Input: part model. Units: mm. Frame: model coordinates. A direction names the side the tool comes from. Give positions to 0.01 mm unless a question says otherwise; leave off trailing zeros. Loops run counter-clockwise (first coordinate to the right, second up) from the corner with the lowest first, then second, coordinate; pieces in that order, holes last. Notation, with made-up numbers: (42.5, 61.5) - (96.5, 61.5) arc R15 cw to (96.5, 69.5) - close; hole circle Ø4 at (9.25, 80.5). An arc over 180 degrees is marked (long way). Answer as a JSON object with one key per item and string values. Group by question number.
(1) Access query for faces 1 (the cylindrical face through (14.13, 1.69, 1.84)), 2 (the flat face through (4.06, -6.66, 5.94)), 3 (the flat face through (4.06, 6.66, -5.94)). Directions: +Z, -Z, +X, -X, +Y, -Y. A direction counts if a zero-diameter tool reaches every point of the face in a straight line with its end or side. Return the directions, or none.
(2) Section query B-B (x = 21). Return loops of the section in (y, z), plus the area to 3 significant figures.
(3) Pin query (flat end, axial travel): P1, Ø4, axis at x = 4, z = 1.5, coming from the -Y side; P2, Ø3.5, axis at y = -0.5, z = -0.5, coming from the +X side; P3, Ø6, axis at x = 17, z = 7.5, coming from the -Y side. Return the tip coordinate at first contact, or that it passes through.
(4) Mould query, pull axis X, two halves, no side actions, for faces 4 (the cylindrical face through (17.666, -8.428, -1.107)), 5 (the flat face through (23, -2, -2)), 6 (the flat face through (13.209, -7, 3)), 7 (the flat face through (0, 0, 0)). Classes: +X half, -X half, draft (parallel to the pull), parting line (faces both ways), or undercut.
(5) Material intervals for L1, parallel to Y at x = 17.75, z = 0; L2, parallel to Y at x = 10.5, z = 0; L3, parallel to X at y = -11, z = 6.75, sorted ascending.
(6) Section query A-A (x = 7.5). Return loops of the section in (y, z).
```python
from build123d import *

# Parameters (mm, degrees)
EXTRUDE_START            = -8
SKETCH_2_R               = 8.5
EXTRUDE_1_DEPTH          = 8
CHAMFER_1_SIZE           = 1
SKETCH_3_R               = 2.5
CUT_EXTRUDE_1_DEPTH      = 18
CUT_EXTRUDE_2_DEPTH      = 18
CUT_EXTRUDE_2_DEPTH_BACK = 8.454068
SKETCH_4_R               = 2.5


with BuildPart() as part:
    # Sketch 1 → 旋转1 (revolve)
    with BuildSketch(Plane.XY, mode=Mode.PRIVATE) as revolve_1_sk:
        Polygon((0, 0), (0, 8.5), (8, 8.5), (8, 13), (11, 13), (11.209265355, 7.3), (13.209265355, 7.3), (13.209265355, 8.5), (23, 8.5), (23, 0), align=None)
    revolve(revolve_1_sk.sketch.rotate(Axis((0, 0, 0), (1, 0, 0)), 90), axis=Axis((0, 0, 0), (1, 0, 0)))

    # 草图2 → 凸台-拉伸1 (add)
    # profile 1 of 7: a face of its own
    with BuildSketch(Plane.ZY.offset(EXTRUDE_START)):
        Polygon((-1.174764966, -9.690972033), (7.805245485, -5.86286232), (8.980010451, 3.828109713), (1.174764966, 9.690972033), (-7.805245485, 5.86286232), (-8.980010451, -3.828109713), align=None)
        Circle(SKETCH_2_R, mode=Mode.SUBTRACT)
    # profile 2 of 7: a face of its own
    with BuildSketch(Plane.ZY.offset(EXTRUDE_START)):
        with BuildLine():
            Line((-7.805245485, 5.86286232), (-8.286430908, 1.893426207))
            ThreePointArc((-8.286430908, 1.893426207), (-6.796266629, 5.104974035), (-4.12702026, 7.430861577))
            Line((-4.12702026, 7.430861577), (-7.805245485, 5.86286232))
        make_face()
    # profile 3 of 7: a face of its own
    with BuildSketch(Plane.ZY.offset(EXTRUDE_START)):
        with BuildLine():
            ThreePointArc((-2.503460259, 8.122972777), (1.022903886, 8.43822657), (4.371804767, 7.289535176))
            Line((4.371804767, 7.289535176), (1.174764966, 9.690972033))
            Line((1.174764966, 9.690972033), (-2.503460259, 8.122972777))
        make_face()
    # profile 4 of 7: a face of its own
    with BuildSketch(Plane.ZY.offset(EXTRUDE_START)):
        with BuildLine():
            ThreePointArc((8.5, 0), (8.499706252, -0.070665642), (8.498825028, -0.141326401))
            Line((8.498825028, -0.141326401), (8.980010451, 3.828109713))
            Line((8.980010451, 3.828109713), (5.78297065, 6.22954657))
            ThreePointArc((5.78297065, 6.22954657), (7.79118895, 3.398142837), (8.5, 0))
        make_face()
    # profile 5 of 7: a face of its own
    with BuildSketch(Plane.ZY.offset(EXTRUDE_START)):
        with BuildLine():
            Line((4.12702026, -7.430861577), (7.805245485, -5.86286232))
            Line((7.805245485, -5.86286232), (8.286430908, -1.893426207))
            ThreePointArc((8.286430908, -1.893426207), (6.796266629, -5.104974035), (4.12702026, -7.430861577))
        make_face()
    # profile 6 of 7: a face of its own
    with BuildSketch(Plane.ZY.offset(EXTRUDE_START)):
        with BuildLine():
            Line((-1.174764966, -9.690972033), (2.503460259, -8.122972777))
            ThreePointArc((2.503460259, -8.122972777), (-1.022903886, -8.43822657), (-4.371804767, -7.289535176))
            Line((-4.371804767, -7.289535176), (-1.174764966, -9.690972033))
        make_face()
    # profile 7 of 7: a face of its own
    with BuildSketch(Plane.ZY.offset(EXTRUDE_START)):
        with BuildLine():
            Line((-8.980010451, -3.828109713), (-5.78297065, -6.22954657))
            ThreePointArc((-5.78297065, -6.22954657), (-7.819170515, -3.333252534), (-8.498825028, 0.141326401))
            Line((-8.498825028, 0.141326401), (-8.980010451, -3.828109713))
        make_face()
    extrude(amount=EXTRUDE_1_DEPTH)

    # 倒角1
    chamfer_1_edges = [part.edges().sort_by_distance(p)[0] for p in [
        (23, 0, -8.5),
    ]]
    chamfer(chamfer_1_edges, length=CHAMFER_1_SIZE)

    # 草图3 → 切除-拉伸1 (cut)
    with BuildSketch(Plane(origin=(23, 0, 0), x_dir=(0, 0, -1), z_dir=(1, 0, 0))):
        Circle(SKETCH_3_R)
    extrude(amount=-CUT_EXTRUDE_1_DEPTH, mode=Mode.SUBTRACT)

    # 草图4 → 切除-拉伸2 (cut, two sides: drawn at the far end of the back side and taken through both)
    with BuildSketch(Plane(origin=(0, -6.759540873, -5.077387708), x_dir=(1, 0, 0), z_dir=(0, -0.7995607799259467, -0.6005851806398588)).offset(-CUT_EXTRUDE_2_DEPTH_BACK)):
        with Locations(Location((4, 0, 0), (0, 0, 66.421821522))):
            Circle(SKETCH_4_R)
    extrude(amount=CUT_EXTRUDE_2_DEPTH + CUT_EXTRUDE_2_DEPTH_BACK, mode=Mode.SUBTRACT)


solid = part.part
```
Recorded:
{
 "1": {"face 1": "+X", "face 2": "+Z, -X, -Y", "face 3": "-Z, -X, +Y"},
 "2": {"outline": "circle Ø17 at (0, 0); hole circle Ø5 at (0, 0)", "area": "207 mm^2"},
 "3": {"P1": "stops at y = -9.4", "P2": "stops at x = 5", "P3": "stops at y = -7.21"},
 "4": {"face 4": "draft", "face 5": "+X half", "face 6": "undercut", "face 7": "-X half"},
 "5": {"L1": "y = -8.5 to -2.5, 2.5 to 8.5", "L2": "y = -13 to -2.5, 2.5 to 13", "L3": "x = 8 to 11"},
 "6": {"outline": "(-9.69, -1.17) - (-7.29, -4.37) arc R8.5 ccw to (-6.23, -5.78) - (-3.83, -8.98) - (0.14, -8.5) arc R8.5 ccw to (1.89, -8.29) - (5.86, -7.81) - (7.43, -4.13) arc R8.5 ccw to (8.12, -2.5) - (9.69, 1.17) - (7.29, 4.37) arc R8.5 ccw to (6.23, 5.78) - (3.83, 8.98) - (-0.14, 8.5) arc R8.5 ccw to (-1.89, 8.29) - (-5.86, 7.81) - (-7.43, 4.13) arc R8.5 ccw to (-8.12, 2.5) - close; hole circle Ø5 at (0, 0)"}
}
